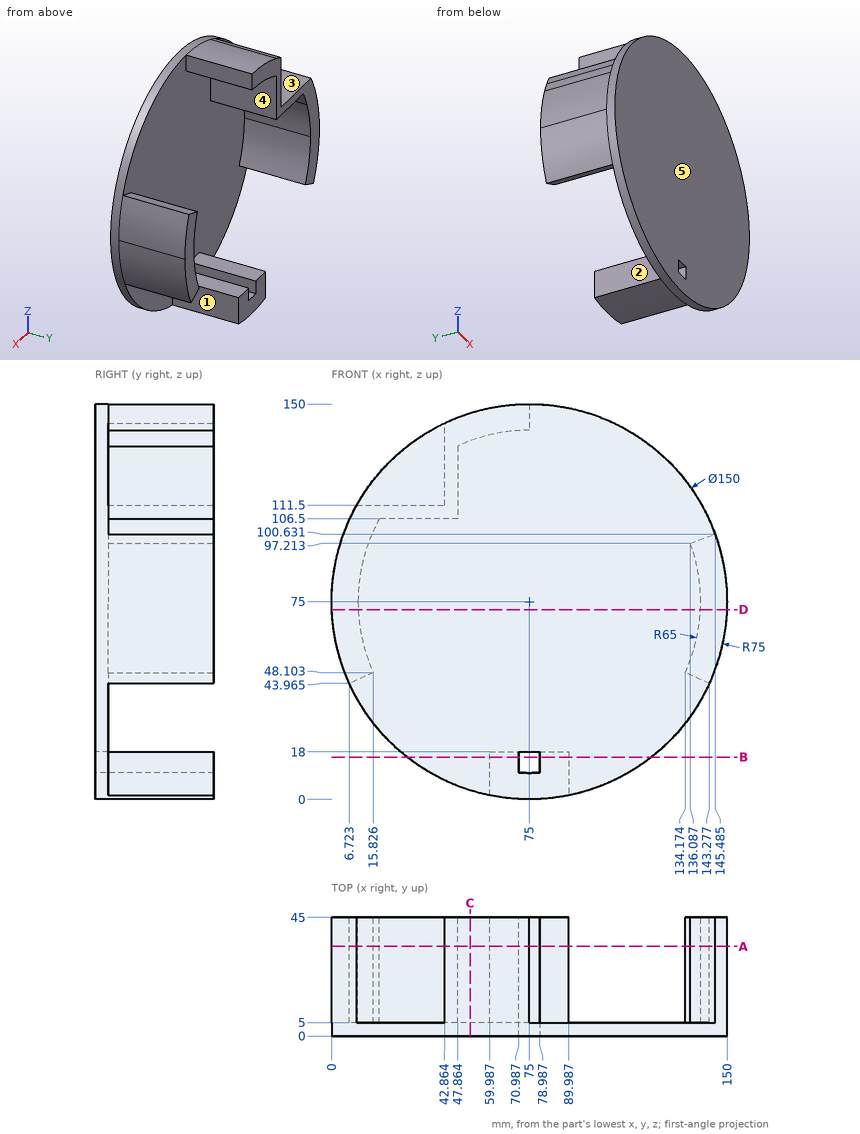
Source: three-view drawing plus pictorial views. Frame: mm from the lowest corner of the part. A direction names the side the tool comes from. Round coordinates to 2 decimals unless told otherwise and drop trailing zeros. Loops run counter-clockwise (first coordinate to the right, second up) from the corner with the lowest first, then second, coordinate; pieces in that order, holes last.
Q1. Section A-A on y = 34. Return loops of the section in (x, z) (1 decimal).
Q2. Section C-C on x = 52.5. Return loops of the section in (y, z) (1 decimal).
Q3. Section B-B on z = 16. Return loops of the section in (x, y).
Q4. Material intervals for L1, parallel to X at y = 42, z = 13; L2, parallel to Y at x = 39, z = 61; L3, parallel to X at y = 12, z = 79, sorted ascending.
Q5. Pin query (flat end, axial travel): P1, Ø2.5, axis at y = 21, z = 13.5, coming from the +X side; P2, Ø9.5, axis at y = 30, z = 131.5, coming from the -X side; P3, Ø25, axis at x = 18, z = 127.5, coming from the +Y side. Return the tip coordinate at first contact, or that it passes through.
Q6. Access query for the marked faces 1, 2, 3, 4 and 5. Directions: +Z, -Z, +X, -X, +Y, -Y. A direction counts if a zero-diameter tool reaches every point of the face in a straight line with its end or side. Return the directions, or none.
Q7. Section D-D on z = 72. Return loops of the section in (x, y).
Evaluation:
1. outline: (6.7, 44) - (15.8, 48.1) arc R65 cw to (18.1, 106.5) - (47.9, 106.5) - (47.9, 134.1) arc R65 cw to (75, 140) - (75, 150) arc R75 ccw to (42.9, 142.8) - (42.9, 111.5) - (9.5, 111.5) arc R75 ccw to start; (60, 1.5) arc R75 ccw to (90, 1.5) - (90, 18) - (79, 18) - (79, 10.1) arc R65 cw to (71, 10.1) - (71, 18) - (60, 18) - close; (134.2, 48.1) - (143.3, 44) arc R75 ccw to (145.5, 100.6) - (136.1, 97.2) arc R65 cw to start
2. outline: (0, 3.5) - (5, 3.5) - (5, 136) - (45, 136) - (45, 146.5) - (0, 146.5) - close
3. outline: (28.7, 0) - (70.99, 0) - (70.99, 45) - (59.99, 45) - (59.99, 5) - (28.7, 5) - close; (78.99, 0) - (121.3, 0) - (121.3, 5) - (89.99, 5) - (89.99, 45) - (78.99, 45) - close
4. L1: x = 59.99 to 70.99, 78.99 to 89.99
4. L2: y = 0 to 5
4. L3: x = 0.11 to 10.12, 139.88 to 149.89
5. P1: stops at x = 89.99
5. P2: stops at x = 42.86
5. P3: stops at y = 5
6. face 1: +Z, -Z, +X, +Y
6. face 2: -Z, -X, +Y
6. face 3: +Z, -X, +Y
6. face 4: -Z, +X, +Y
6. face 5: +Z, -Z, +X, -X, -Y
7. outline: (0.06, 0) - (149.94, 0) - (149.94, 45) - (139.93, 45) - (139.93, 5) - (10.07, 5) - (10.07, 45) - (0.06, 45) - close
